Check sheet for the modelled part. Datum: model origin and axes. Units: mm. A direction names the side the tool comes from. Give positions to 0.01 mm unless a question says otherwise; leave off trailing zeros. Loops run counter-clockwise (first coordinate to the right, second up) from the corner with the lowest first, then second, coordinate; pieces in that order, holes last. Notation, with made-up numbers: (-22, 6) - (-7, 6) arc R25 ccw to (-7, 39) - close; hole circle Ø9 at (65.5, 21.5). An arc over 180 degrees is marked (long way). Use one line per item in the form item = value.
from build123d import *

# Parameters (mm, degrees)
SKETCH033_W             = 36
SKETCH033_H             = 41
SKETCH033_R             = 1.65
EXTRUDE035_DEPTH        = 2
SKETCH039_W             = 14.242
SKETCH039_H             = 2.925
EXTRUDE039_DEPTH        = 0.5
LINK007_PLACEMENT_ANGLE = 65
SKETCH040_W             = 40
SKETCH040_H             = 38
EXTRUDE041_DEPTH        = 2
EXTRUDE040_DEPTH        = 4
SKETCH041_W             = 40
SKETCH041_H             = 45.78385
EXTRUDE042_DEPTH        = 2
SKETCH042_W             = 34
SKETCH042_H             = 18.982178
EXTRUDE043_DEPTH        = 4
SKETCH043_W             = 40
SKETCH043_H             = 5
EXTRUDE044_DEPTH        = 4


with BuildPart() as extrude_displaycase_front:
    # Sketch033 → Extrude035 (new body)
    with BuildSketch(Plane.XY):
        with Locations((13.635, 13)):
            Rectangle(SKETCH033_W, SKETCH033_H)
        with Locations((3, 30.31)):
            Circle(SKETCH033_R, mode=Mode.SUBTRACT)
        with Locations((24.27, 30.31)):
            Circle(SKETCH033_R, mode=Mode.SUBTRACT)
        with Locations((3, -2)):
            Circle(SKETCH033_R, mode=Mode.SUBTRACT)
        with Locations((24.27, -2)):
            Circle(SKETCH033_R, mode=Mode.SUBTRACT)
        Polygon((27.37, 23.21), (27.37, 3.51), (-0.1, 3.51), (-0.1, 23.21), (6.514, 23.21), (6.514, 26.135), (20.756, 26.135), (20.756, 23.21), align=None, mode=Mode.SUBTRACT)
    extrude(amount=-EXTRUDE035_DEPTH)


with BuildPart() as fusion_displaycase_front001:
    # Sketch039 → Extrude039 (new body)
    with BuildSketch(Plane.XY):
        with Locations((13.635, 24.6725)):
            Rectangle(SKETCH039_W, SKETCH039_H)
    extrude(amount=-EXTRUDE039_DEPTH)

    # Fusion012: union Extrude_DisplayCase_Front
    add(extrude_displaycase_front.part)


with BuildPart() as fusion_displaycase_front001_1:
    # Link007 placement: moved
    add(fusion_displaycase_front001.part.moved(Location((6.5, 3.2, 12))).rotate(Axis((6.5, 3.2, 12), (1, 0, 0)), LINK007_PLACEMENT_ANGLE))


with BuildPart() as extrude_displaycase_bottom:
    # Sketch040 → Extrude041 (new body)
    with BuildSketch(Plane.XY):
        Polygon((40, 40), (0, 40), (-2.12132, 40), (-2.12132, -2.12132), (42.12132, -2.12132), (42.12132, 40), align=None)
        with Locations((20, 19)):
            Rectangle(SKETCH040_W, SKETCH040_H, mode=Mode.SUBTRACT)
    extrude(amount=EXTRUDE041_DEPTH)


with BuildPart() as extrude_displaycase_side:
    # Sketch032 → Extrude040 (new body)
    with BuildSketch(Plane.YZ):
        Polygon((0, 5), (19.017822, 45.78385), (40, 45.78385), (40, 5), (40, 0), (0, 0), align=None)
    extrude(amount=EXTRUDE040_DEPTH)


with BuildPart() as extrude_displaycase_side001:
    # Link006 base: copy of Extrude_DisplayCase_Side
    add(extrude_displaycase_side.part)


with BuildPart() as extrude_displaycase_side001_1:
    # Link006 placement: moved
    add(extrude_displaycase_side001.part.moved(Location((36, 0, 0))))


with BuildPart() as extrude_displaycase_back:
    # Sketch041 → Extrude042 (new body)
    with BuildSketch(Plane.XZ):
        with Locations((20, 22.891925)):
            Rectangle(SKETCH041_W, SKETCH041_H)
    extrude(amount=EXTRUDE042_DEPTH)


with BuildPart() as extrude_displaycase_back_1:
    # Extrude042 placement: moved
    add(extrude_displaycase_back.part.moved(Location((0, 40, 0))))


with BuildPart() as extrude_displaycase_top:
    # Sketch042 → Extrude043 (new body)
    with BuildSketch(Plane.XY):
        with Locations((21, 28.508911)):
            Rectangle(SKETCH042_W, SKETCH042_H)
    extrude(amount=-EXTRUDE043_DEPTH)


with BuildPart() as extrude_displaycase_top_1:
    # Extrude043 placement: moved
    add(extrude_displaycase_top.part.moved(Location((0, 0, 45.78385))))


with BuildPart() as extrude_displaycase_frontbottom:
    # Sketch043 → Extrude044 (new body)
    with BuildSketch(Plane.XZ):
        with Locations((20, 2.5)):
            Rectangle(SKETCH043_W, SKETCH043_H)
    extrude(amount=-EXTRUDE044_DEPTH)


with BuildPart() as cut_displaycase:
    # Fusion013 base: copy of Extrude_DisplayCase_Side
    add(extrude_displaycase_side.part)

    # Fusion013: union Extrude_DisplayCase_Bottom, Extrude_DisplayCase_Side001, Extrude_DisplayCase_Back, Extrude_DisplayCase_Top, Extrude_DisplayCase_FrontBottom
    add(extrude_displaycase_bottom.part)
    add(extrude_displaycase_side001_1.part)
    add(extrude_displaycase_back_1.part)
    add(extrude_displaycase_top_1.part)
    add(extrude_displaycase_frontbottom.part)

    # Cut010: cut Fusion_DisplayCase_Front001
    add(fusion_displaycase_front001_1.part, mode=Mode.SUBTRACT)


with BuildPart() as cut_displaycase_1:
    # Cut010 placement: moved
    add(cut_displaycase.part.moved(Location((5, 5, 28))))


solid = cut_displaycase_1.part
Item 1: Section check D-D on y = 30.5. Record the boundary of the cut face in (x, z), then the cut area to 3 significant figures.
Answer block:
outline = (2.88, 28) - (9, 28) - (9, 69.78) - (41, 69.78) - (41, 28) - (47.12, 28) - (47.12, 30) - (45, 30) - (45, 73.78) - (5, 73.78) - (5, 30) - (2.88, 30) - close
area = 503 mm2
Item 2: Section check C-C on x = 42. Record the boundary of the cut face in (y, z).
Answer block:
outline = (2.88, 28) - (45, 28) - (45, 73.78) - (24.02, 73.78) - (22.41, 70.34) - (24.17, 69.52) - (6.84, 32.36) - (5.08, 33.18) - (5, 33) - (5, 30) - (2.88, 30) - close
Item 3: Access from +Z, -Z, +X, -X, +Y, -Y to the whole of each face (thin tool, end or side, straight path). Record for faces 4 (the face through (25, 5, 31)), 5 (the face through (5, 30, 52)), 6 (the face through (24.88, 6.15, 32.68)).
Answer block:
face_4 = +Z, +X, -X, -Y
face_5 = +Z, -X, +Y, -Y
face_6 = +Z
Item 4: Thickness scan on L1, parallel to X at y = 16.5, z = 33; L2, parallel to Y at x = 32, z = 47.5; L3, parallel to Z at x = 33.5, y = 42.5. Record the ranges inside material, lowest first.
Answer block:
L1 = 5 to 9, 41 to 45
L2 = 43 to 45
L3 = 69.78 to 73.78
Item 5: Mould release check, pull along Z, two halves, no side actions. Record for faces 1 (the face through (45, 30, 52)), 2 (the face through (25, 8, 33)), 3 (the face through (42.05, 23.28, 69.93)): released by +Z, released by -Z, zero draft, split by the parting line, or undercut.
Answer block:
face_1 = zero draft
face_2 = released by +Z
face_3 = undercut
Item 6: Section check B-B on x = 15. Record the boundary of the cut face in (y, z).
Answer block:
outline = (2.88, 28) - (9, 28) - (9, 33) - (7.14, 33) - (6.84, 32.36) - (5.47, 33) - (5, 33) - (5, 30) - (2.88, 30) - close; (24.02, 69.78) - (43, 69.78) - (43, 28) - (45, 28) - (45, 73.78) - (24.02, 73.78) - close
Item 7: Gauge pin test, flat ends, axial feed: P1, Ø3, axis at x = 20, z = 71, coming from the -Y side; P2, Ø18, axis at y = 21, z = 60.5, coming from the +X side; P3, Ø9.5, axis at x = 18, z = 46, coming from the -Y side; P4, Ø10, axis at y = 9, z = 58, coming from the +X side. Record the tip position at first contact, or that the pin passes through.
Answer block:
P1 = 24.02
P2 = 45
P3 = 43
P4 = through
Item 8: Section check A-A on y = 14. Record the boundary of the cut face in (x, z) (3 decimals).
Answer block:
outline = (2.879, 28) - (9, 28) - (9, 47.706) - (7.135, 47.706) - (7.135, 52.301) - (5, 52.301) - (5, 30) - (2.879, 30) - close; (41, 28) - (47.121, 28) - (47.121, 30) - (45, 30) - (45, 52.301) - (43.135, 52.301) - (43.135, 47.706) - (41, 47.706) - close
